from build123d import *

# Parameters (mm, degrees)
SKETCH1_R           = 3.175
BOSS_EXTRUDE1_DEPTH = 114.3
SKETCH2_R           = 3.175
BOSS_EXTRUDE2_DEPTH = 50.8
SKETCH3_R           = 1.5875
CUT_EXTRUDE1_DEPTH  = 115.3


with BuildPart() as part:
    # Sketch1 → Boss-Extrude1 (new body)
    with BuildSketch(Plane(origin=(0, 0, 0), x_dir=(1, 0, 0), z_dir=(0, 1, 0))):
        Circle(SKETCH1_R)
    extrude(amount=BOSS_EXTRUDE1_DEPTH)

    # Sketch2 → Boss-Extrude2 (add)
    with BuildSketch(Plane.XY):
        with Locations((0, 25.4)):
            Circle(SKETCH2_R)
    extrude(amount=BOSS_EXTRUDE2_DEPTH)

    # Sketch3 → Cut-Extrude1 (cut, through all)
    with BuildSketch(Plane(origin=(0, 0, 0), x_dir=(1, 0, 0), z_dir=(0, 1, 0))):
        with Locations((0, -44.45)):
            Circle(SKETCH3_R)
    extrude(amount=CUT_EXTRUDE1_DEPTH, mode=Mode.SUBTRACT)


solid = part.part
Work out the finished part from the listing and answer in its coordinate system (mm). A direction names the side the tool comes from. Give positions to 0.01 mm unless a question says otherwise; leave off trailing zeros. Loops run counter-clockwise (first coordinate to the right, second up) from the corner with the lowest first, then second, coordinate; pieces in that order, holes last. Notation, with made-up numbers: (-18.5, 3.5) - (-2.5, 3.5) arc R16 cw to (-2.5, 7.5) - close; hole circle Ø6 at (49, -33). An arc over 180 degrees is marked (long way). Answer in a Markdown table with one row per item. Add a question column.
Q1. The part is cut by section D-D (z = 1.5). Determine the outline of the cut face in (x, y) (3 decimals), and give its area (3 significant figures).
Q2. Determine the mould class of faces 1 (the flat face through (0, 25, 50.8)), 2 (the cylindrical face through (1.466, 25.356, 45.058)), 3 (the flat face through (0, 114.3, 0)) for opening direction Z: released by +Z, released by -Z, zero draft, split by the parting line, or undercut.
Q3. The part is cut by section A-A (x = 0). Determine the outline of the cut face in (y, z) (1 decimal).
Q4. A tool of negligible diameter and unlimited length cuts with its end or side. For faces 4 (the cylindrical face through (-3.17, 25.54, 25.04)), 5 (the flat face through (0, 0, 0)), from which of +Z, -Z, +X, -X, +Y, -Y can it reach the whole face along a straight path? Write none if from no direction.
Q5. Consider line 1 along Z through (x, y) = (0, 26.25) (1 decimal); line 2 along X through (y, z) = (24, 44); line 3 along X through (y, z) = (25, 44.45). Determine where each line is inside the solid, lowest interval first.
Q6. The part is cut by section C-C (y = 99). Determine the outline of the cut face in (x, z) (3 decimals).
Q7. Each of these flat-tipped pins is pushed along its axis until it touches: P1, Ø1, axis at x = 2.5, y = 37, coming from the +Z side; P2, Ø3, axis at x = -0.5, y = 53, coming from the +Z side (3 decimals). Where does it stop, or does it pass through?
Solution:
| question | item | result |
|---|---|---|
| 1 | outline | (-2.798, 0) - (2.798, 0) - (2.798, 23.9) arc R3.175 ccw to (2.798, 26.9) - (2.798, 114.3) - (-2.798, 114.3) - (-2.798, 26.9) arc R3.175 ccw to (-2.798, 23.9) - close |
| 1 | area | 641 mm² |
| 2 | face 1 | released by +Z |
| 2 | face 2 | undercut |
| 2 | face 3 | zero draft |
| 3 | outline | (0, -3.2) - (114.3, -3.2) - (114.3, 3.2) - (28.6, 3.2) - (28.6, 42.9) - (22.2, 42.9) - (22.2, 3.2) - (0, 3.2) - close; (22.2, 46) - (28.6, 46) - (28.6, 50.8) - (22.2, 50.8) - close |
| 4 | face 4 | +Z |
| 4 | face 5 | +Z, -Z, +X, -X, -Y |
| 5 | line 1 | z = -3.2 to 42.9, 46 to 50.8 |
| 5 | line 2 | x = -2.85 to -1.52, 1.52 to 2.85 |
| 5 | line 3 | x = -3.15 to -1.59, 1.59 to 3.15 |
| 6 | outline | circle Ø6.35 at (0, 0) |
| 7 | P1 | stops at z = 2.47 |
| 7 | P2 | stops at z = 3.175 |
